Autodesk Inventor part; units mm, degrees
ref_plane "YZ Plane" through (0, 0, 0) normal (1, 0, 0) x (0, 1, 0)
ref_plane "XZ Plane" through (0, 0, 0) normal (0, 1, 0) x (-1, 0, 0)
ref_plane "XY Plane" through (0, 0, 0) normal (0, 0, 1) x (1, 0, 0)
sketch "Boceto1" plane through (0, 0, 0) normal (0, 1, 0) x (-1, 0, 0)
  line L0 (0, 0) -> (220.8, 0)
  line L1 (220.8, 0) -> (220.8, -220.8)
  line L2 (220.8, -220.8) -> (0, -220.8)
  line L3 (0, -220.8) -> (0, 0)
  line L4 (211.6, -211.6) -> (211.6, -147.2)
  line L5 (211.6, -9.2) -> (156.4, -9.2)
  line L6 (9.2, -211.6) -> (73.6, -211.6)
  line L7 (73.6, -211.6) -> (73.6, -209.3)
  line L8 (75.9, -71.3) -> (211.6, -71.3)
  line L9 (149.5, -211.6) -> (149.5, -75.9)
  line L10 (211.6, -9.2) -> (211.6, -71.3)
  line L11 (211.6, -75.9) -> (211.6, -82.8)
  line L12 (211.6, -211.6) -> (211.6, -75.9)
  line L13 (211.6, -71.3) -> (211.6, -9.2)
  line L14 (75.9, -75.9) -> (144.9, -75.9)
  line L15 (149.5, -75.9) -> (211.6, -75.9)
  line L16 (9.2, -149.5) -> (144.9, -149.5)
  line L17 (144.9, -211.6) -> (144.9, -149.5)
  line L18 (144.9, -144.9) -> (144.9, -75.9)
  line L19 (71.3, -144.9) -> (71.3, -9.2)
  line L20 (9.2, -144.9) -> (71.3, -144.9)
  line L21 (75.9, -144.9) -> (144.9, -144.9)
  line L22 (75.9, -144.9) -> (75.9, -75.9)
  line L23 (75.9, -71.3) -> (75.9, -9.2)
  line L24 (211.6, -9.2) -> (75.9, -9.2)
  line L25 (71.3, -9.2) -> (9.2, -9.2)
  line L26 (9.2, -9.2) -> (9.2, -144.9)
  line L27 (9.2, -149.5) -> (9.2, -211.6)
  line L28 (9.2, -211.6) -> (144.9, -211.6)
  line L29 (149.5, -211.6) -> (211.6, -211.6)
  dimension "d0" = 220.8
  dimension "d1" = 220.8
extrude "Extrusión1" add sketch "Boceto1" along normal blind 4
chamfer "Chaflán1" distance 4 angle 45 4 edges at (-220.8, 4, -110.4) (-110.4, 4, 0) (0, 4, -110.4) (-110.4, 4, -220.8) measured on face at (-121.9, 4, -217.7333)
sketch "Boceto2" plane through (0, 0, 0) normal (0, -1, 0) x (1, 0, 0)
  line L0 (-216.8, -4) -> (-216.8, -216.8)
  line L1 (0, -220.8) -> (-220.8, -220.8)
  line L2 (0, 0) -> (0, -220.8)
  line L3 (-220.8, 0) -> (0, 0)
  line L4 (-220.8, -220.8) -> (-220.8, 0)
  line L5 (-9.2, -211.6) -> (-9.2, -149.5)
  line L6 (-144.9, -211.6) -> (-9.2, -211.6)
  line L7 (-144.9, -149.5) -> (-144.9, -211.6)
  line L8 (-9.2, -149.5) -> (-144.9, -149.5)
  line L9 (-71.3, -144.9) -> (-9.2, -144.9)
  line L10 (-71.3, -9.2) -> (-71.3, -144.9)
  line L11 (-9.2, -9.2) -> (-71.3, -9.2)
  line L12 (-9.2, -144.9) -> (-9.2, -9.2)
  line L13 (-75.9, -144.9) -> (-75.9, -75.9)
  line L14 (-144.9, -144.9) -> (-75.9, -144.9)
  line L15 (-144.9, -75.9) -> (-144.9, -144.9)
  line L16 (-75.9, -75.9) -> (-144.9, -75.9)
  line L17 (-149.5, -75.9) -> (-211.6, -75.9)
  line L18 (-149.5, -211.6) -> (-149.5, -75.9)
  line L19 (-211.6, -211.6) -> (-149.5, -211.6)
  line L20 (-211.6, -75.9) -> (-211.6, -211.6)
  line L21 (-75.9, -71.3) -> (-75.9, -9.2)
  line L22 (-211.6, -71.3) -> (-75.9, -71.3)
  line L23 (-211.6, -9.2) -> (-211.6, -71.3)
  line L24 (-75.9, -9.2) -> (-211.6, -9.2)
  circle A0 centre (-110.4, -110.4) radius 34.5
  circle A1 centre (-110.4, -110.4) radius 22.8
  dimension "d31" = 45.6
extrude "Extrusión2" add sketch "Boceto2" against normal blind 4 contours L14 A0 L13 | A0 L16 L13 | A0 | L14 L15 A0 | A0 L15 L16
properties part number "Lampara2base"
Source: CAD feature listing. Evaluate the final solid. Frame: model axes, mm. Give positions to 0.01 mm unless a question says otherwise; leave off trailing zeros. Order: outer loops, then holes, each group sorted by start corner. A loop starts at its lowest first (then second) coordinate and runs counter-clockwise, first axis right, second up.
(1) Contact query for flat-ended pins moving along their axis: P1, Ø2, axis at x = -54, y = 1.5, coming from the -Z side; P2, Ø2, axis at y = 3, z = -115.5, coming from the -X side; P3, Ø1, axis at y = 1, z = -158.5, coming from the +X side. Output: stop coordinate, or through.
(2) Section query A-A (x = -110.4). State how many separate pieces and enclosed holes the cut face has, plus the area to 3 significant figures.
(3) Material intervals for line 1 along Z through (x, y) = (-161, 3.3); line 2 along X through (y, z) = (0.65, -95); line 3 along Z through (x, y) = (-110.4, 1.3), sorted ascending.
(4) Pull-direction query (X, two-part tool) for faces 1 (the face through (-88.653, 1.972, -103.551)), 2 (the face through (-110, 4, -134)); classes: +X half, -X half, draft (parallel to the pull), parting line (faces both ways), or undercut.
(5) Section query D-D (y = 3.4). Return the cut outline in (x, z).
Outcome:
1. P1: stops at z = -220.3
1. P2: stops at x = -218.8
1. P3: stops at x = -0.5
2. separate pieces: 4
2. enclosed holes: 0
2. area: 188 mm2
3. line 1: z = -217.5 to -211.6, -75.9 to -71.3, -9.2 to -3.3
3. line 2: x = -220.15 to -211.6, -149.5 to -127.21, -93.59 to -71.3, -9.2 to -0.65
3. line 3: z = -219.5 to -211.6, -149.5 to -133.2, -87.6 to -71.3, -9.2 to -1.3
4. face 1: undercut
4. face 2: draft
5. outline: (-217.4, -217.4) - (-3.4, -217.4) - (-3.4, -3.4) - (-217.4, -3.4) - close; hole (-211.6, -211.6) - (-149.5, -211.6) - (-149.5, -75.9) - (-211.6, -75.9) - close; hole (-211.6, -71.3) - (-75.9, -71.3) - (-75.9, -9.2) - (-211.6, -9.2) - close; hole (-144.9, -211.6) - (-9.2, -211.6) - (-9.2, -149.5) - (-144.9, -149.5) - close; hole circle Ø45.6 at (-110.4, -110.4); hole (-71.3, -144.9) - (-9.2, -144.9) - (-9.2, -9.2) - (-71.3, -9.2) - close
